```python
from build123d import *

# Parameters (mm, degrees)
F0_W     = 50
F0_H     = 50
F1_DEPTH = 35
F4_DEPTH = 74.8112648726
F6_SIZE  = 3
F7_R     = 0.5
F8_R     = 7.5
F8_R_2   = 5
F9_DEPTH = 13


# Not quite as in the source:
# - a pattern or mirror of a feature is missing from the dataset's text; its kind, count and spacing are read off the source's solid


with BuildPart() as f1:
    # F0 (on Top) → F1 (new body)
    with BuildSketch(Plane.XY):
        Rectangle(F0_W, F0_H)
    extrude(amount=F1_DEPTH)

    # F3 (on face) → F4 (cut)
    with BuildSketch(Plane(origin=(25, -25, 0), x_dir=(-0.7071067812, -0.7071067812, 0), z_dir=(-0.7071067812, 0.7071067812, 0))):
        Polygon((27.3553390593, 20), (21.8957855453, 35), (12.8148925733, 35), (7.3553390593, 20), align=None)
    f4 = extrude(amount=F4_DEPTH, mode=Mode.SUBTRACT)

    # F4_copies: F4 across plane
    add(f4.mirror(Plane(origin=(0, 0, 0), x_dir=(0.7071067812, -0.7071067812, 0), z_dir=(0.7071067812, 0.7071067812, 0))), mode=Mode.SUBTRACT)

    # F6
    f6_edges = [f1.edges().sort_by_distance(p)[0] for p in [
        (25, 0, 0),
        (0, -25, 0),
        (-25, 0, 0),
        (0, 25, 0),
        (25, -25, 17.5),
        (-25, -25, 17.5),
        (-25, 25, 17.5),
        (25, 25, 17.5),
    ]]
    chamfer(f6_edges, length=F6_SIZE)

    # F7
    f7_edges = [f1.edges().sort_by_distance(p)[0] for p in [
        (-15.482658, -15.482658, 35),
        (-9.061497, -9.061497, 35),
        (9.061497, 9.061497, 35),
        (15.482658, 15.482658, 35),
    ]]
    fillet(f7_edges, radius=F7_R)

    # F8 (on face) → F9 (cut)
    with BuildSketch(Plane.XY.offset(35)):
        with Locations((-14.8947280353, 15.1347092162)):
            Circle(F8_R)
        with Locations((-14.8947280353, 15.1347092162)):
            Circle(F8_R_2, mode=Mode.SUBTRACT)
    extrude(amount=-F9_DEPTH, mode=Mode.SUBTRACT)


solid = f1.part
```
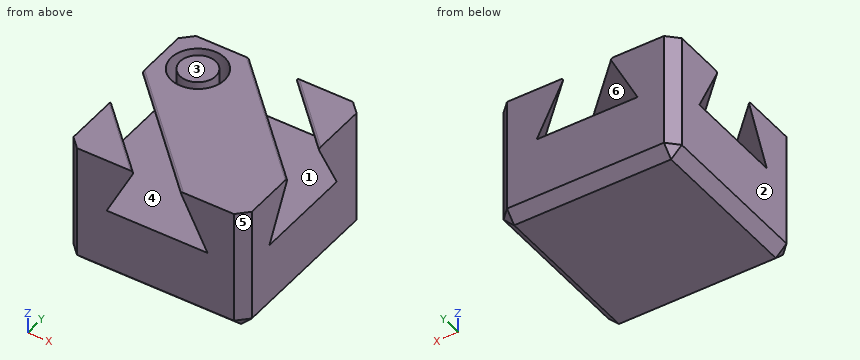
Here's how the part is built. I have some questions about the finished solid (model axes, mm). Face numbers are marked on the shaded views. A direction names the side the tool comes from. Give positions to 0.01 mm unless a question says otherwise; leave off trailing zeros. Write each loop counter-clockwise with the first axis right and the second up, starting at its lowest first coordinate (ties: lowest second). Pieces come first, ordered by that corner, then holes. Notation, with made-up numbers: (17.25, 61.5) -> (47.25, 61.5) arc R19 cw to (47.25, 72.5) -> close; hole circle Ø9 at (44.5, 38). An arc over 180 degrees is marked (long way). Use one line per item in the form item = value.
1) On a 3-axis mill with a long thin cutter (end or side, diameter ignored), from which of +Z, -Z, +X, -X, +Y, -Y can I reach the whole of each face in a straight line? I mean the marked faces 1 and 2. Say none if no direction works.
Verdict:
face_1 = none
face_2 = +Z, -Z, -X, +Y, -Y
2) If I drill on L1, parallel to Y at x = -19.5, z = 28.5; L2, parallel to Z at x = -2, y = -20; L3, parallel to X at y = 15.5, z = 32, over which ranges is the centre line in solid material (lowest first)? Write a range as [from, to].
Verdict:
L1 = [-25, -14.81], [4.72, 9.22], [13.19, 17.08], [21.05, 25]
L2 = [0, 20]
L3 = [-25, -22.39], [-19.88, -9.91], [-7.4, 1.08], [17.01, 25]
3) Suppose I cut it at B-B (z = 32). Please give me the cut outline in (x, y), and give its area (3 significant figures).
Verdict:
outline = (-25, -22) -> (-22, -25) -> (-7.51, -25) -> (-25, -7.51) -> close; (-25, 8.42) -> (8.42, -25) -> (22, -25) -> (25, -22) -> (25, -8.42) -> (-8.42, 25) -> (-22, 25) -> (-25, 22) -> close; circle Ø10 at (-14.89, 15.13); (7.51, 25) -> (25, 7.51) -> (25, 22) -> (22, 25) -> close; hole circle Ø15 at (-14.89, 15.13)
area = 1,570 mm2
4) I'm going to push flat-ended pins straight in: pin 1 (3 mm diameter, centred on y = 5.5, z = 30, fed in from +X); pin 2 (3 mm diameter, centred on x = 1.5, z = 26, fed in from +Y). Where does each tip first touch, or does it pass through?
Verdict:
pin_1 = 11.74
pin_2 = 13.68
5) We'd pull the mould along Y, two halves only. Please class the marked faces 3, 4, 5 and 6: +Y half, -Y half, draft (parallel to the pull), parting line (faces both ways), or undercut.
Verdict:
face_3 = draft
face_4 = undercut
face_5 = -Y half
face_6 = undercut
6) Suppose I cut it at A-A (z = 24.5). Please give me the cut outline in (x, y), and give its area (3 significant figures).
Verdict:
outline = (-25, -22) -> (-22, -25) -> (-11.37, -25) -> (-25, -11.37) -> close; (-25, 12.28) -> (12.28, -25) -> (22, -25) -> (25, -22) -> (25, -12.28) -> (-12.28, 25) -> (-22, 25) -> (-25, 22) -> close; circle Ø10 at (-14.89, 15.13); (11.37, 25) -> (25, 11.37) -> (25, 22) -> (22, 25) -> close; hole circle Ø15 at (-14.89, 15.13)
area = 1,180 mm2
